Check sheet for the drawn part. Datum: minimum x, y, z corner. Units: mm. A direction names the side the tool comes from. Coordinates: 2 decimals unless noted, no trailing zeros. Loops run counter-clockwise (first coordinate to the right, second up) from the corner with the lowest first, then second, coordinate; pieces in that order, holes last. Notation, with made-up numbers: (37.25, 42) -> (85.25, 42) arc R5 ccw to (85.25, 47) -> close; hole circle Ø5 at (41, -34). An arc over 180 degrees is marked (long way). Use CSV: the item, a comma, the result in double quotes. Start each with the question number.
1. Sectioned sample at C-C, the plane z = 5. Record the cut outline in (x, y).
2. Release check for a two-part mould opening along Y. For the marked faces 3, 4 and 5 record: pulls with the +Y half, pulls with the -Y half, needs draft (parallel to the pull), parting line crosses it, or undercut.
3. Sectioned sample at A-A, the plane x = 10. Record the cut outline in (y, z).
4. Set-up check for the marked faces 1 and 2: record each of +Z, -Z, +X, -X, +Y, -Y from which the full face is reachable in a straight line by a thin tool's end or side.
5. Gauge pin test, flat end, axial feed: pin 1 (9 mm diameter, centred on x = 10, y = 20, fed in from +Z). Record the tip position at first contact, or that the pin passes through.
6. Sectioned sample at D-D, the plane x = 25. Record the cut outline in (y, z).
7. Sectioned sample at B-B, the plane y = 5. Record the cut outline in (x, z).
8. Thickness scan on L1, parallel to X at y = 20, z = 1.4; L2, parallel to Y at x = 40, z = 2.1; L3, parallel to X at y = 5, z = 7.75. Record the ranges inside material, lowest first.
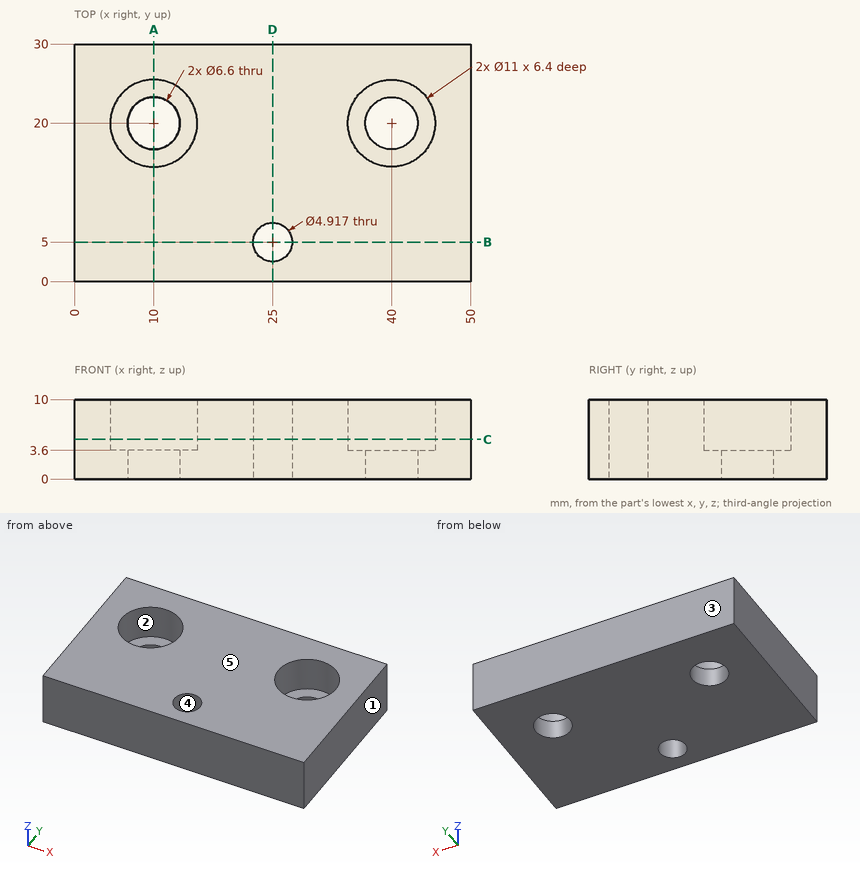
Completed:
1,outline,"(0, 0) -> (50, 0) -> (50, 30) -> (0, 30) -> close; hole circle Ø11 at (10, 20); hole circle Ø4.92 at (25, 5); hole circle Ø11 at (40, 20)"
2,face 3,"pulls with the +Y half"
2,face 4,"undercut"
2,face 5,"needs draft"
3,outline,"(0, 0) -> (16.7, 0) -> (16.7, 3.6) -> (14.5, 3.6) -> (14.5, 10) -> (0, 10) -> close; (23.3, 0) -> (30, 0) -> (30, 10) -> (25.5, 10) -> (25.5, 3.6) -> (23.3, 3.6) -> close"
4,face 1,"+Z, -Z, +X, +Y, -Y"
4,face 2,"+Z"
5,pin 1,"z = 3.6"
6,outline,"(0, 0) -> (2.54, 0) -> (2.54, 10) -> (0, 10) -> close; (7.46, 0) -> (30, 0) -> (30, 10) -> (7.46, 10) -> close"
7,outline,"(0, 0) -> (22.54, 0) -> (22.54, 10) -> (0, 10) -> close; (27.46, 0) -> (50, 0) -> (50, 10) -> (27.46, 10) -> close"
8,L1,"0 to 6.7, 13.3 to 36.7, 43.3 to 50"
8,L2,"0 to 16.7, 23.3 to 30"
8,L3,"0 to 22.54, 27.46 to 50"
